Source: CAD feature listing. Evaluate the final solid. Frame: model axes, mm. A direction names the side the tool comes from. Give positions to 0.01 mm unless a question says otherwise; leave off trailing zeros. Order: outer loops, then holes, each group sorted by start corner. A loop starts at its lowest first (then second) coordinate and runs counter-clockwise, first axis right, second up.
from build123d import *

# Parameters (mm, degrees)
SKETCH_1_W                  = 55
SKETCH_1_H                  = 60
EXTRUDE_1_DEPTH             = 16.5
HOLE_WIZARD_3_6_3_6_1_D     = 3.6
HOLE_WIZARD_3_6_3_6_1_DEPTH = 25
HOLE_WIZARD_3_6_3_6_1_TIP   = 1.081549114
HOLE_WIZARD_M2_5_1_D        = 2.05
HOLE_WIZARD_M2_5_1_DEPTH    = 14
HOLE_WIZARD_M2_5_1_TIP      = 0.615882135
SKETCH_8_W                  = 35
SKETCH_8_H                  = 20.4
CUT_EXTRUDE_1_DEPTH         = 44.914690025
CUT_EXTRUDE_START           = 2.5
SKETCH_9_W                  = 20
SKETCH_9_H                  = 6
CUT_EXTRUDE_2_DEPTH         = 42.414690025
SHELL_START                 = 1.8
SHELL_1_DEPTH               = 14.7
EXTRUDE_2_DEPTH             = 7
SKETCH_16_R                 = 3
CUT_EXTRUDE_4_DEPTH         = 12
CUT_EXTRUDE_5_DEPTH         = 47.120928005
CUT_EXTRUDE_5_DEPTH_BACK    = 47.120928005
SKETCH_17_R                 = 6
FILLET_1_R                  = 0.5
FILLET_2_R                  = 0.5
HOLE_WIZARD_1_AT_2_COUNT    = 2
HOLE_WIZARD_1_AT_2_PITCH    = 27.5
HOLE_WIZARD_1_AT_3_COUNT    = 2
HOLE_WIZARD_1_AT_3_PITCH    = 61.846584384
HOLE_WIZARD_1_AT_4_COUNT    = 2
HOLE_WIZARD_1_AT_4_PITCH    = 48
SKETCH_21_W                 = 80
SKETCH_21_H                 = 100
EXTRUDE_3_DEPTH             = 7
HOLE_WIZARD_2_D             = 4.5
HOLE_WIZARD_2_CBORE_D       = 8
HOLE_WIZARD_2_CBORE_DEPTH   = 4.6
SKETCH_24_R                 = 8.656208536
EXTRUDE_4_DEPTH             = 4
FILLET_3_R                  = 5
HOLE_WIZARD_M6_2_D          = 5
HOLE_WIZARD_M6_2_DEPTH      = 15
HOLE_WIZARD_M6_2_TIP        = 1.502151548


# Read off the part's stored shape, not the designer's step: 抽壳1
with BuildPart() as part:
    # 草图1 → 凸台-拉伸1 (new body)
    with BuildSketch(Plane.XY):
        Rectangle(SKETCH_1_W, SKETCH_1_H)
    extrude(amount=EXTRUDE_1_DEPTH)

    # Ø3.6 (3.6) 直径孔1
    with Locations(Plane.XY.offset(16.5)):
        with Locations((-24, 21.5), (24, 21.5), (24, -6), (-15, -26.5)):
            Hole(HOLE_WIZARD_3_6_3_6_1_D / 2, depth=HOLE_WIZARD_3_6_3_6_1_DEPTH)
            with Locations((0, 0, -(HOLE_WIZARD_3_6_3_6_1_DEPTH + HOLE_WIZARD_3_6_3_6_1_TIP / 2))):  # 118° drill point
                Cone(0, HOLE_WIZARD_3_6_3_6_1_D / 2, HOLE_WIZARD_3_6_3_6_1_TIP, mode=Mode.SUBTRACT)

    # M2.5 螺纹孔1
    with Locations(Plane.XY.offset(16.5)):
        with Locations((-24, 26.5), (24, 26.5), (24, -1), (-22.5, -26.5)):
            Hole(HOLE_WIZARD_M2_5_1_D / 2, depth=HOLE_WIZARD_M2_5_1_DEPTH)
            with Locations((0, 0, -(HOLE_WIZARD_M2_5_1_DEPTH + HOLE_WIZARD_M2_5_1_TIP / 2))):  # 118° drill point
                Cone(0, HOLE_WIZARD_M2_5_1_D / 2, HOLE_WIZARD_M2_5_1_TIP, mode=Mode.SUBTRACT)

    # 草图8 → 切除-拉伸1 (cut, through all)
    with BuildSketch(Plane.XY.offset(16.5)):
        with Locations((10, -19.8)):
            Rectangle(SKETCH_8_W, SKETCH_8_H)
    extrude(amount=-CUT_EXTRUDE_1_DEPTH, mode=Mode.SUBTRACT)

    # 草图9 → 切除-拉伸2 (cut, through all)
    with BuildSketch(Plane(origin=(0, 0, 16.5), x_dir=(-1, 0, 0), z_dir=(0, 0, -1)).offset(CUT_EXTRUDE_START)):
        with Locations((17.5, -27)):
            Rectangle(SKETCH_9_W, SKETCH_9_H)
    extrude(amount=CUT_EXTRUDE_2_DEPTH, mode=Mode.SUBTRACT)

    # 抽壳1 outline → 抽壳1 (cut)
    with BuildSketch(Plane.XY.offset(SHELL_START)):
        with BuildLine():
            ThreePointArc((-21.743758657, 28.2), (-21.182110509, 26.299690696), (-22.006919283, 24.4979375))
            ThreePointArc((-22.006919283, 24.4979375), (-20.910890356, 19.651378458), (-25.7, 18.326673669))
            Line((-25.7, 18.326673669), (-25.7, -22.2))
            Line((-25.7, -22.2), (-9.3, -22.2))
            Line((-9.3, -22.2), (-9.3, -7.8))
            Line((-9.3, -7.8), (20.882308546, -7.8))
            ThreePointArc((20.882308546, -7.8), (20.494996561, -5.178446051), (22.006919283, -3.0020625))
            ThreePointArc((22.006919283, -3.0020625), (21.865811165, 0.8509087), (25.7, 1.256241343))
            Line((25.7, 1.256241343), (25.7, 18.326673669))
            ThreePointArc((25.7, 18.326673669), (20.910890356, 19.651378458), (22.006919283, 24.4979375))
            ThreePointArc((22.006919283, 24.4979375), (21.182110509, 26.299690696), (21.743758657, 28.2))
            Line((21.743758657, 28.2), (-21.743758657, 28.2))
        make_face()
    extrude(amount=SHELL_1_DEPTH, mode=Mode.SUBTRACT)

    # 草图16 → 切除-拉伸4 (cut)
    with BuildSketch(Plane(origin=(-7.5, 0, 0), x_dir=(0, 0, -1), z_dir=(1, 0, 0))):
        with Locations(Location((-8, -18, 0), (0, 0, 90))):
            Circle(SKETCH_16_R)
    extrude(amount=-CUT_EXTRUDE_4_DEPTH, mode=Mode.SUBTRACT)


with BuildPart() as body_2:
    # 草图10 → 凸台-拉伸2 (new body)
    with BuildSketch(Plane.XY.offset(16.5)):
        Polygon((-27.5, -30), (-7.5, -30), (-7.5, -9.6), (27.5, -9.6), (27.5, 30), (-27.5, 30), align=None)
    extrude(amount=EXTRUDE_2_DEPTH)


with BuildPart() as cut_extrude_5_tool:
    # 草图17 → 切除-拉伸5 (new, two sides: drawn at the far end of the back side and taken through both)
    with BuildSketch(Plane.XY.offset(1.8).offset(-CUT_EXTRUDE_5_DEPTH_BACK)):
        with Locations((6.5, 9.5)):
            Circle(SKETCH_17_R)
    extrude(amount=CUT_EXTRUDE_5_DEPTH + CUT_EXTRUDE_5_DEPTH_BACK)


with BuildPart() as part_1:
    add(part.part)

    # 切除-拉伸5: cut by cut_extrude_5_tool
    add(cut_extrude_5_tool.part, mode=Mode.SUBTRACT)

    # 圆角1
    fillet_1_edges = [part_1.edges().sort_by_distance(p)[0] for p in [
        (-27.5, 3, 0),
        (0, 30, 0),
        (27.5, 10.2, 0),
        (27.5, -9.6, 8.25),
        (-7.5, -16.8, 0),
        (10, -9.6, 0),
        (-7.5, -9.6, 8.25),
        (-7.5, -30, 15.25),
        (-27.5, -30, 15.25),
        (-27.5, 30, 8.25),
        (27.5, 30, 8.25),
        (-17.5, -24, 0),
        (-7.5, -24, 7),
        (-27.5, -24, 7),
    ]]
    fillet(fillet_1_edges, radius=FILLET_1_R)


with BuildPart() as body_2_1:
    add(body_2.part)

    # 切除-拉伸5: cut by cut_extrude_5_tool
    add(cut_extrude_5_tool.part, mode=Mode.SUBTRACT)

    # 圆角2
    fillet_2_edges = [body_2_1.edges().sort_by_distance(p)[0] for p in [
        (-27.5, 30, 20),
        (27.5, 30, 20),
        (27.5, -9.6, 20),
        (-7.5, -9.6, 20),
        (-7.5, -30, 20),
        (-27.5, -30, 20),
    ]]
    fillet(fillet_2_edges, radius=FILLET_2_R)

    # 草图20 → 打孔尺寸(%根据)内六角圆柱头螺钉的类型1 (revolve, cut)
    with BuildSketch(Plane(origin=(24, 21.5, 16.5), x_dir=(0, 1, 0), z_dir=(1, 0, 0))):
        Polygon((0, 0), (0, 7), (2.25, 7), (2.25, 4.6), (4, 4.6), (4, 0), align=None)
    hole_wizard_1 = revolve(axis=Axis((24, 21.5, 10.15), (0, 0, 1)), mode=Mode.SUBTRACT)

    # 打孔尺寸(%根据)内六角圆柱头螺钉的类型1 at 2: 打孔尺寸(%根据)内六角圆柱头螺钉的类型1 ×2
    with Locations(*[(0, -i * HOLE_WIZARD_1_AT_2_PITCH, 0) for i in range(1, HOLE_WIZARD_1_AT_2_COUNT)]):
        add(hole_wizard_1, mode=Mode.SUBTRACT)

    # 打孔尺寸(%根据)内六角圆柱头螺钉的类型1 at 3: 打孔尺寸(%根据)内六角圆柱头螺钉的类型1 ×2
    with Locations(*[Vector(-0.6305926250944656, -0.7761140001162656, 0) * (i * HOLE_WIZARD_1_AT_3_PITCH) for i in range(1, HOLE_WIZARD_1_AT_3_COUNT)]):
        add(hole_wizard_1, mode=Mode.SUBTRACT)

    # 打孔尺寸(%根据)内六角圆柱头螺钉的类型1 at 4: 打孔尺寸(%根据)内六角圆柱头螺钉的类型1 ×2
    with Locations(*[(-i * HOLE_WIZARD_1_AT_4_PITCH, 0, 0) for i in range(1, HOLE_WIZARD_1_AT_4_COUNT)]):
        add(hole_wizard_1, mode=Mode.SUBTRACT)

    # 草图21 → 凸台-拉伸3 (add)
    with BuildSketch(Plane.XY.offset(23.5)):
        Rectangle(SKETCH_21_W, SKETCH_21_H)
        with BuildLine():
            Line((-27, -30), (-8, -30))
            ThreePointArc((-8, -30), (-7.646446609, -29.853553391), (-7.5, -29.5))
            Line((-7.5, -29.5), (-7.5, -10.1))
            ThreePointArc((-7.5, -10.1), (-7.353553391, -9.746446609), (-7, -9.6))
            Line((-7, -9.6), (27, -9.6))
            ThreePointArc((27, -9.6), (27.353553391, -9.453553391), (27.5, -9.1))
            Line((27.5, -9.1), (27.5, 29.5))
            ThreePointArc((27.5, 29.5), (27.353553391, 29.853553391), (27, 30))
            Line((27, 30), (-27, 30))
            ThreePointArc((-27, 30), (-27.353553391, 29.853553391), (-27.5, 29.5))
            Line((-27.5, 29.5), (-27.5, -29.5))
            ThreePointArc((-27.5, -29.5), (-27.353553391, -29.853553391), (-27, -30))
        make_face(mode=Mode.SUBTRACT)
    extrude(amount=-EXTRUDE_3_DEPTH)

    # 打孔尺寸(%根据)内六角圆柱头螺钉的类型2 (through all)
    with Locations(Plane(origin=(0, 0, 16.5), x_dir=(-1, 0, 0), z_dir=(0, 0, -1))):
        with Locations((-24, 21.5), (-24, -6), (15, -26.5), (24, 21.5)):
            CounterBoreHole(HOLE_WIZARD_2_D / 2, HOLE_WIZARD_2_CBORE_D / 2, HOLE_WIZARD_2_CBORE_DEPTH)

    # 草图24 → 凸台-拉伸4 (add)
    with BuildSketch(Plane(origin=(0, 0, 16.5), x_dir=(-1, 0, 0), z_dir=(0, 0, -1))):
        with Locations((-6.5, 9.5)):
            Circle(SKETCH_24_R)
    extrude(amount=-EXTRUDE_4_DEPTH)

    # 圆角3
    fillet_3_edges = [body_2_1.edges().sort_by_distance(p)[0] for p in [
        (-40, 50, 20),
        (-40, -50, 20),
        (40, -50, 20),
        (40, 50, 20),
    ]]
    fillet(fillet_3_edges, radius=FILLET_3_R)

    # M6 螺纹孔2
    with Locations(Plane.XY.offset(23.5)):
        with Locations((33, 41), (-33, 41), (-33, -41), (33, -41)):
            Hole(HOLE_WIZARD_M6_2_D / 2, depth=HOLE_WIZARD_M6_2_DEPTH)
            with Locations((0, 0, -(HOLE_WIZARD_M6_2_DEPTH + HOLE_WIZARD_M6_2_TIP / 2))):  # 118° drill point
                Cone(0, HOLE_WIZARD_M6_2_D / 2, HOLE_WIZARD_M6_2_TIP, mode=Mode.SUBTRACT)


solid = body_2_1.part
(1) Section C-C, the plane x = -15. Return loops of the section in (y, z).
(2) Section D-D, the plane y = -41. Return loops of the section in (x, z), plus the area to 3 significant figures.
(3) Line query: line 1 along Y through (x, z) = (33, 18.75); line 2 along X through (y, z) = (21.5, 22.4); line 3 along Y through (x, z) = (-24, 21.75). Output: solid intervals per line, ascending.
(4) Access query for faces 5 (the flat face through (7, 10, 20.5)), 6 (the flat face through (-1, 1, 23.5)). Directions: +Z, -Z, +X, -X, +Y, -Y. A direction counts if a zero-diameter tool reaches every point of the face in a straight line with its end or side. Return the directions, or none.
(5) Pin query (flat end, axial travel): pin 1 Ø5 at (x, y) = (-15, -26.5) entering from +Z; pin 2 Ø6 at (x, y) = (4, 8) entering from +Z. Return the tip coordinate at first contact, or that it passes through.
(6) Section A-A, the plane y = -26.5. Return loops of the section in (x, z), plus the area to 3 significant figures.
(7) Draft query along X for faces 1 (the flat face through (-1, 1, 16.5)), 2 (the cylindrical face through (-15.099, -28.748, 22.283)), 3 (the cylindrical face through (-39, 48, 20)), 4 (the flat face through (40, -1, 20)). Return one class per face: +X half, -X half, draft (parallel to the pull), parting line (faces both ways), or undercut.
(8) Section B-B, the plane x = 33. Return loops of the section in (y, z).
Checks:
1. outline: (-50, 16.5) - (-30.5, 16.5) - (-30.5, 21.1) - (-28.75, 21.1) - (-28.75, 23.5) - (-50, 23.5) - close; (-24.25, 21.1) - (-22.5, 21.1) - (-22.5, 16.5) - (50, 16.5) - (50, 23.5) - (-24.25, 23.5) - close
2. outline: (-40, 16.5) - (-35.5, 16.5) - (-35.5, 23.5) - (-40, 23.5) - close; (-30.5, 16.5) - (30.5, 16.5) - (30.5, 23.5) - (-30.5, 23.5) - close; (35.5, 16.5) - (40, 16.5) - (40, 23.5) - (35.5, 23.5) - close
2. area: 490 mm2
3. line 1: y = -50 to -43.5, -38.5 to 38.5, 43.5 to 50
3. line 2: x = -40 to -26.25, -21.75 to 21.75, 26.25 to 40
3. line 3: y = -50 to 19.25, 23.75 to 50
4. face 5: +Z
4. face 6: +Z, +X, -X, +Y, -Y
5. pin 1: stops at z = 23.5
5. pin 2: stops at z = 20.5
6. outline: (-40, 16.5) - (-19, 16.5) - (-19, 21.1) - (-17.25, 21.1) - (-17.25, 23.5) - (-40, 23.5) - close; (-12.75, 21.1) - (-11, 21.1) - (-11, 16.5) - (40, 16.5) - (40, 23.5) - (-12.75, 23.5) - close
6. area: 512 mm2
7. face 1: draft
7. face 2: undercut
7. face 3: -X half
7. face 4: +X half
8. outline: (-50, 16.5) - (-43.5, 16.5) - (-43.5, 23.5) - (-50, 23.5) - close; (-38.5, 16.5) - (38.5, 16.5) - (38.5, 23.5) - (-38.5, 23.5) - close; (43.5, 16.5) - (50, 16.5) - (50, 23.5) - (43.5, 23.5) - close
